Check sheet for the drawn part. Datum: minimum x, y, z corner. Units: mm. Give positions to 0.01 mm unless a question says otherwise; leave off trailing zeros. Write each loop counter-clockwise with the first axis right and the second up, starting at its lowest first coordinate (ties: lowest second). Pieces come first, ordered by that corner, then holes. Notation, with made-up numbers: M 3,55.25 L 46,55.25 A21 ccw 46,88.25 Z; hole C -3,-9.5 d6. An arc over 180 degrees is marked long. Use CSV: the item, a comma, the result in double quotes. Start each with the question number.
1. Cross-section at C-C, the plane z = 2.15. State how many separate pieces and enclosed holes the cut face has, and give its area (3 significant figures).
2. Cross-section at A-A, the plane y = 10. Enter the section's corners in (x, z).
3. Depth check by flat-ended pin: P1, Ø1.5, axis at x = 107.5, z = 1, coming from the +Y side; P2, Ø0.9, axis at x = 4, z = 1, coming from the +Y side; P3, Ø0.9, axis at y = 107.5, z = 1, coming from the -X side; P4, Ø4.5, axis at x = 10, y = 10, coming from the +Z side. Enter the tip coordinate at first touch or a pass-through.
4. Cross-section at B-B, the plane x = 88. Enter the section's corners in (y, z), and give its area (3 significant figures).
5. Scan lines: line 1 (Y direction, x = 10, z = 0.9); line 2 (Y direction, x = 42, z = 1.35). Record each from-to range of solid material in increasing order.
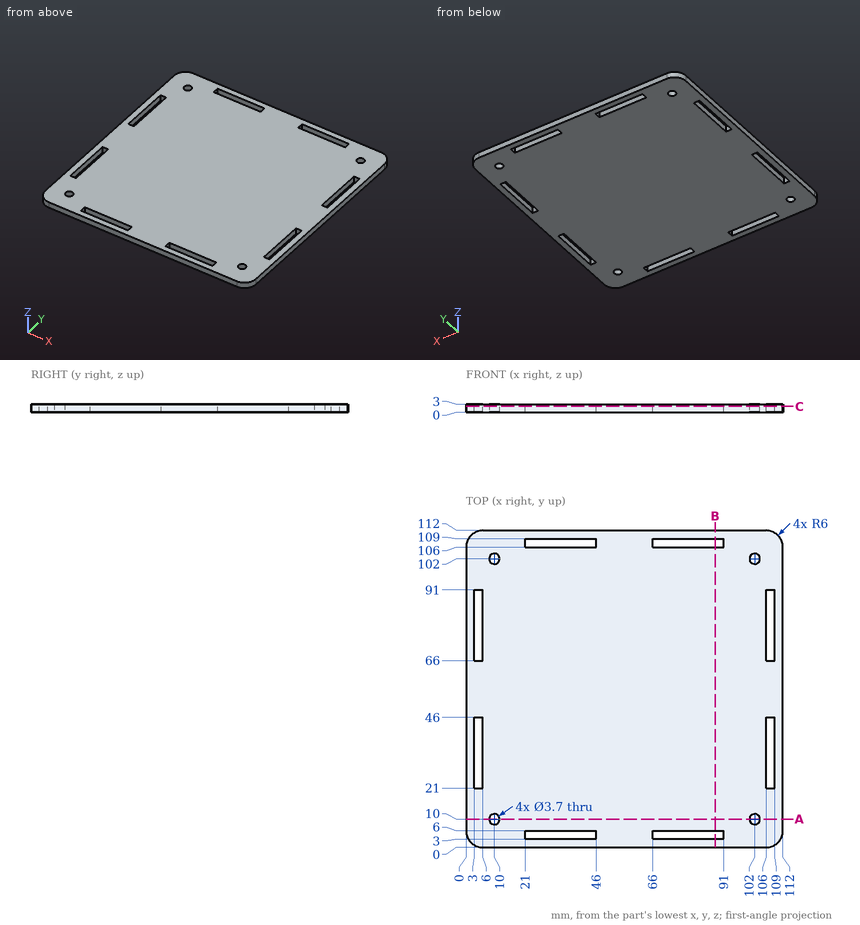
Worked answers:
1,separate pieces,"1"
1,enclosed holes,"12"
1,area,"11,900 mm^2"
2,outline,"M 0,0 L 8.15,0 L 8.15,3 L 0,3 Z; M 11.85,0 L 100.15,0 L 100.15,3 L 11.85,3 Z; M 103.85,0 L 112,0 L 112,3 L 103.85,3 Z"
3,P1,"stops at y = 111.95"
3,P2,"stops at y = 111.8"
3,P3,"stops at x = 0.09"
3,P4,"stops at z = 3"
4,outline,"M 0,0 L 3,0 L 3,3 L 0,3 Z; M 6,0 L 106,0 L 106,3 L 6,3 Z; M 109,0 L 112,0 L 112,3 L 109,3 Z"
4,area,"318 mm^2"
5,line 1,"y = 0 to 8.15, 11.85 to 100.15, 103.85 to 112"
5,line 2,"y = 0 to 3, 6 to 106, 109 to 112"
